```python
from build123d import *

# Parameters (mm, degrees)
F1_DEPTH  = 5.842
F2_DEPTH  = 5.08
F3_W      = 18.542
F3_H      = 5.08
F4_DEPTH  = 35.56
F5_W      = 18.542
F5_H      = 5.08
F6_DEPTH  = 58.42
F8_DEPTH  = 2.54
F9_DEPTH  = 2.54
F7_W      = 19.7188566824
F7_H      = 3.81
F10_DEPTH = 25.4
F11_DEPTH = 3.81
F12_DEPTH = 5.08
F13_DEPTH = 7.62
F14_W     = 18.542
F14_H     = 5.08
F15_DEPTH = 127
F16_R     = 5.07999
F18_DEPTH = 2.54
F19_W     = 5.08
F19_H     = 12.7
F20_DEPTH = 5.08


# Not quite as in the source:
# - two fillets or chamfers of one size are made in one step
# - a fillet or chamfer is up to 0.001 mm smaller than in the source, because OpenCascade refuses the exact size


with BuildPart() as f1:
    # F0 (on Top) → F1 (new body)
    with BuildSketch(Plane.XY):
        Polygon((-9.271, 43.18), (-9.271, 0), (-6.731, 0), (-6.731, 12.7), (6.731, 12.7), (6.731, 0), (9.271, 0), (9.271, 43.18), align=None)
    extrude(amount=F1_DEPTH)

    # F2 (add): a face of the model
    f2_faces = [f1.faces().sort_by_distance(p)[0] for p in [
        (0, 43.18, 2.921),
    ]]
    extrude(f2_faces, amount=F2_DEPTH)

    # F3 (on face) → F4 (join)
    with BuildSketch(Plane.XY.offset(5.842)):
        with Locations((0, 45.72)):
            Rectangle(F3_W, F3_H)
    extrude(amount=F4_DEPTH)

    # F5 (on face) → F6 (join)
    with BuildSketch(Plane.XZ.offset(-43.18)):
        with Locations((0, 38.862)):
            Rectangle(F5_W, F5_H)
    extrude(amount=F6_DEPTH)

    # F8 (add): a face of the model
    f8_faces = [f1.faces().sort_by_distance(p)[0] for p in [
        (-9.271, 0.7580485211, 2.921),
    ]]
    extrude(f8_faces, amount=F8_DEPTH)

    # F9 (add): a face of the model
    f9_faces = [f1.faces().sort_by_distance(p)[0] for p in [
        (9.271, 0.7580485211, 2.921),
    ]]
    extrude(f9_faces, amount=F9_DEPTH)

    # F7 (on face) → F10 (cut)
    with BuildSketch(Plane.XY.offset(41.402)):
        with BuildLine():
            ThreePointArc((3.5898566824, -0.127), (3.9436831489, -1.0504404137), (4.064, -2.032))
            ThreePointArc((4.064, -2.032), (3.9436831489, -3.0135595863), (3.5898566824, -3.937))
            Line((3.5898566824, -3.937), (9.271, -3.937))
            Line((9.271, -3.937), (9.271, -0.127))
            Line((9.271, -0.127), (3.5898566824, -0.127))
        make_face()
        with BuildLine():
            Line((3.5898566824, -3.937), (3.5898566824, -0.127))
            ThreePointArc((3.5898566824, -0.127), (-4.064, -2.032), (3.5898566824, -3.937))
        make_face()
        with BuildLine():
            ThreePointArc((3.5898566824, -3.937), (3.9436831489, -3.0135595863), (4.064, -2.032))
            ThreePointArc((4.064, -2.032), (3.9436831489, -1.0504404137), (3.5898566824, -0.127))
            Line((3.5898566824, -0.127), (3.5898566824, -3.937))
        make_face()
        with Locations((19.1304283412, -2.032)):
            Rectangle(F7_W, F7_H)
    extrude(amount=-F10_DEPTH, mode=Mode.SUBTRACT)

    # F11 (add): a face of the model
    f11_faces = [f1.faces().sort_by_distance(p)[0] for p in [
        (0, 27.2669507324, 0),
    ]]
    extrude(f11_faces, amount=F11_DEPTH)

    # F12 (cut): a face of the model
    f12_faces = [f1.faces().sort_by_distance(p)[0] for p in [
        (0, 12.7, 1.016),
    ]]
    extrude(f12_faces, amount=-F12_DEPTH, mode=Mode.SUBTRACT)

    # F13 (add): a face of the model
    f13_faces = [f1.faces().sort_by_distance(p)[0] for p in [
        (0, 48.26, 18.796),
    ]]
    extrude(f13_faces, amount=F13_DEPTH)

    # F14 (on face) → F15 (cut)
    with BuildSketch(Plane.XY.offset(41.402)):
        with Locations((0, 50.8)):
            Rectangle(F14_W, F14_H)
    extrude(amount=-F15_DEPTH, mode=Mode.SUBTRACT)

    # F16 (radius 5.08 in the source; OpenCascade refuses exactly that, so slightly less here)
    f16_edges = [f1.edges().sort_by_distance(p)[0] for p in [
        (9.271, 53.34, 18.796),
        (-9.271, 53.34, 18.796),
        (-11.811, 55.88, 18.796),
        (-11.811, 43.18, 21.082),
        (11.811, 43.18, 21.082),
        (11.811, 55.88, 18.796),
    ]]
    fillet(f16_edges, radius=F16_R)

    # F18 (add): a face of the model
    f18_faces = [f1.faces().sort_by_distance(p)[0] for p in [
        (0, 48.26, 18.796),
    ]]
    extrude(f18_faces, amount=F18_DEPTH)

    # F19 (on face) → F20 (cut)
    with BuildSketch(Plane(origin=(0, 55.88, 0), x_dir=(-1, 0, 0), z_dir=(0, 1, 0))):
        with Locations((0.127, 19.812)):
            Rectangle(F19_W, F19_H)
    extrude(amount=-F20_DEPTH, mode=Mode.SUBTRACT)


solid = f1.part
```
Input: part model. Units: mm. Frame: model coordinates. A direction names the side the tool comes from. Give positions to 0.01 mm unless a question says otherwise; leave off trailing zeros. Loops run counter-clockwise (first coordinate to the right, second up) from the corner with the lowest first, then second, coordinate; pieces in that order, holes last. Notation, with made-up numbers: (-36, 13) -> (-11, 13) arc R13 ccw to (-11, 37) -> close; hole circle Ø11 at (21.25, 46.5). An arc over 180 degrees is marked (long way). Use a Markdown table: item, result.
Q1. Section query C-C, the plane z = 38. Return the cut outline in (x, y).
Entries:
| item | result |
|---|---|
| outline | (-11.81, -15.24) -> (11.81, -15.24) -> (11.81, -3.94) -> (3.59, -3.94) arc R4.06 cw (long way) to (3.59, -0.13) -> (11.81, -0.13) -> (11.81, 50.8) arc R5.08 ccw to (6.73, 55.88) -> (-6.73, 55.88) arc R5.08 ccw to (-11.81, 50.8) -> close; hole (-8.59, 50.8) -> (8.59, 50.8) arc R5.08 ccw to (4.19, 53.34) -> (-4.19, 53.34) arc R5.08 ccw to start |
Q2. Section query A-A, the plane y = 9. Return the cut outline in (x, z), plus the area to 3 significant figures.
Entries:
| item | result |
|---|---|
| outline | (-11.81, -3.81) -> (-6.73, -3.81) -> (-6.73, 5.84) -> (-11.81, 5.84) -> close; (-11.81, 36.32) -> (11.81, 36.32) -> (11.81, 41.4) -> (-11.81, 41.4) -> close; (6.73, -3.81) -> (11.81, -3.81) -> (11.81, 5.84) -> (6.73, 5.84) -> close |
| area | 218 mm² |
Q3. Section query D-D, the plane z = 15.5. Return the cut outline in (x, y), plus the area to 3 significant figures.
Entries:
| item | result |
|---|---|
| outline | (-11.81, 48.26) arc R5.08 ccw to (-6.73, 43.18) -> (6.73, 43.18) arc R5.08 ccw to (11.81, 48.26) -> (11.81, 50.8) arc R5.08 ccw to (6.73, 55.88) -> (2.41, 55.88) -> (2.41, 53.34) -> (4.19, 53.34) arc R5.08 cw to (8.59, 50.8) -> (-8.59, 50.8) arc R5.08 cw to (-4.19, 53.34) -> (-2.67, 53.34) -> (-2.67, 55.88) -> (-6.73, 55.88) arc R5.08 ccw to (-11.81, 50.8) -> close |
| area | 228 mm² |
Q4. Access query for faces 4 (the flat face through (0, 43.18, 21)), 5 (the flat face through (-9, 0, 1)), 6 (the flat face through (3, 53.34, 19)), 7 (the flat face through (6.731, 9, 1)), 8 (the flat face through (0, 55, 26.162)). Directions: +Z, -Z, +X, -X, +Y, -Y. A direction counts if a zero-diameter tool reaches every point of the face in a straight line with its end or side. Return the directions, or none.
Entries:
| item | result |
|---|---|
| face 4 | +X, -X, -Y |
| face 5 | -Z, +X, -X, -Y |
| face 6 | +Z, -Z |
| face 7 | -Z, -Y |
| face 8 | +Y |
Q5. First-contact query: P1, Ø9.5, axis at x = 0, y = -2.032, coming from the -Z side; P2, Ø2, axis at y = 54.5, z = 22.5, coming from the -X side; P3, Ø7.5, axis at x = -0.5, z = 1, coming from the -Y side; P4, Ø10, axis at x = 0.5, z = 24, coming from the +Y side. Flat tips, straight axial feed; report the tip coordinate or a pass-through.
Entries:
| item | result |
|---|---|
| P1 | stops at z = 36.32 |
| P2 | stops at x = -11.03 |
| P3 | stops at y = 17.78 |
| P4 | stops at y = 55.88 |
Q6. Section query B-B, the plane x = 0. Return the cut outline in (y, z).
Entries:
| item | result |
|---|---|
| outline | (-15.24, 36.32) -> (-6.1, 36.32) -> (-6.1, 41.4) -> (-15.24, 41.4) -> close; (2.03, 36.32) -> (43.18, 36.32) -> (43.18, 5.84) -> (17.78, 5.84) -> (17.78, -3.81) -> (50.8, -3.81) -> (50.8, 41.4) -> (2.03, 41.4) -> close; (53.34, -3.81) -> (55.88, -3.81) -> (55.88, 13.46) -> (53.34, 13.46) -> close; (53.34, 26.16) -> (55.88, 26.16) -> (55.88, 41.4) -> (53.34, 41.4) -> close |
Q7. Pull-direction query (Z, two-part tool) for faces 1 (the flat face through (0, 24, 5.842)), 2 (the flat face through (0, 28, -3.81)), 3 (the flat face through (-6.731, 9, 1)); classes: pulls with the +Z half, pulls with the -Z half, needs draft (parallel to the pull), parting line crosses it, or undercut.
Entries:
| item | result |
|---|---|
| face 1 | undercut |
| face 2 | pulls with the -Z half |
| face 3 | needs draft |
Q8. Ray query, probe 1 along Y at (x, z) = (0, 39.5); probe 2 along X at (y, z) = (5, 0.5); probe 3 along Y at (x, z) = (4, 0.5). Return the intervals inside material, ascending. Write a range as from..to.
Entries:
| item | result |
|---|---|
| probe 1 | y = -15.24..-6.1, 2.03..50.8, 53.34..55.88 |
| probe 2 | x = -11.81..-6.73, 6.73..11.81 |
| probe 3 | y = 17.78..50.8, 53.34..55.88 |
